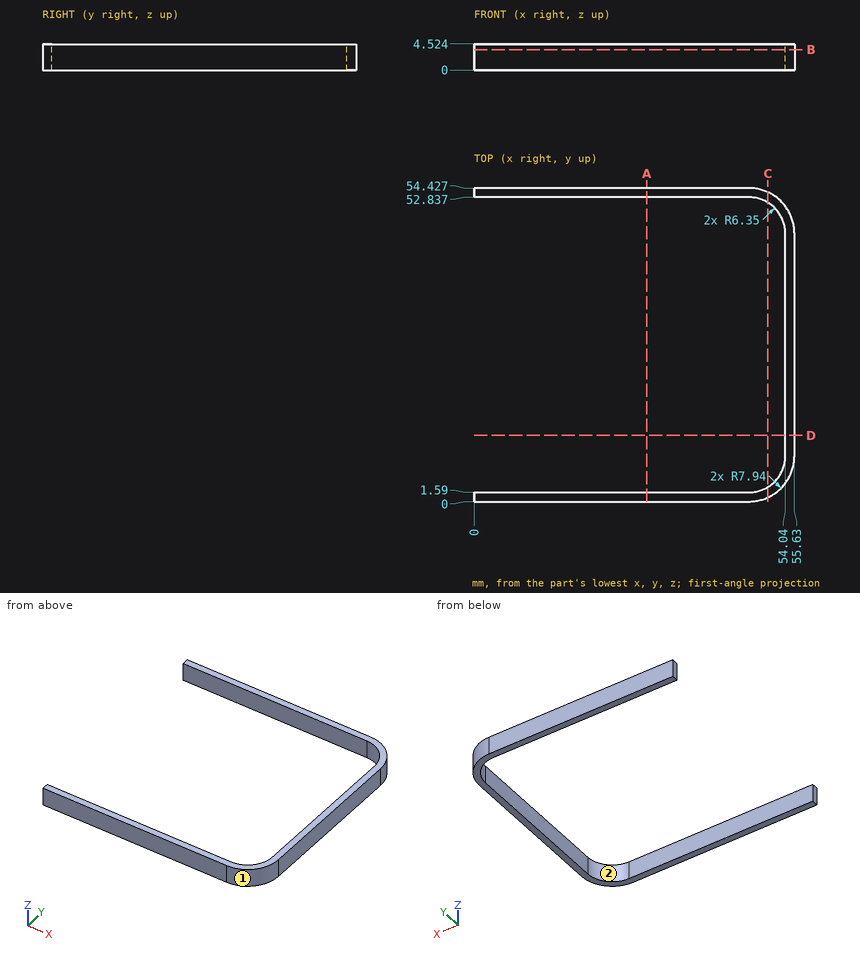
Design review of the part shown in the three views and the two pictorial views. Dimensions are in mm from the part's minimum x, y and z. Give positions to 0.01 mm unless a question says otherwise; leave off trailing zeros. Loops run counter-clockwise (first coordinate to the right, second up) from the corner with the lowest first, then second, coordinate; pieces in that order, holes last. Notation, with made-up numbers: M -27,-37 L -7,-37 A25 cw -7,-11 Z; hole C 12,12 d4. An arc over 180 degrees is marked long. Answer as a JSON object with one key per item and string values.
Item 1: We need section B-B (z = 3.55). State the section outline as (x, y) points.
Output values:
{"outline": "M 0,0 L 47.69,0 A7.94 ccw 55.63,7.94 L 55.63,46.49 A7.94 ccw 47.69,54.43 L 0,54.43 L 0,52.84 L 47.69,52.84 A6.35 cw 54.04,46.49 L 54.04,7.94 A6.35 cw 47.69,1.59 L 0,1.59 Z"}
Item 2: For P1, Ø2.5, axis at x = 14.5, z = 3, coming from the -Y side, flat-tipped, find the tip position at first contact; note if it passes through.
Output values:
{"P1": "stops at y = 0"}
Item 3: Mouldability with a two-part tool opening along Y and no side actions: class the marked faces 1 and 2 as pulls with the +Y half, pulls with the -Y half, needs draft (parallel to the pull), parting line crosses it, or undercut.
Output values:
{"face 1": "pulls with the -Y half", "face 2": "undercut"}
Item 4: We need section D-D (y = 11.5). State the section outline as (x, z) points.
Output values:
{"outline": "M 54.04,0 L 55.63,0 L 55.63,4.52 L 54.04,4.52 Z"}
Item 5: We need section A-A (x = 30). State the section outline as (y, z) points.
Output values:
{"outline": "M 0,0 L 1.59,0 L 1.59,4.52 L 0,4.52 Z; M 52.84,0 L 54.43,0 L 54.43,4.52 L 52.84,4.52 Z"}
Item 6: Wall thickness on line 1 along Y through (x, z) = (8.5, 2.3); line 2 along X through (y, z) = (43, 1.5); line 3 along Y through (x, z) = (49, 1.7): over which ranges is each line inside the solid? List them lowest first.
Output values:
{"line 1": "y = 0 to 1.59, 52.84 to 54.43", "line 2": "x = 54.04 to 55.63", "line 3": "y = 0.11 to 1.73, 52.7 to 54.32"}
Item 7: We need section C-C (x = 51). State the section outline as (y, z) points.
Output values:
{"outline": "M 0.72,0 L 2.52,0 L 2.52,4.52 L 0.72,4.52 Z; M 51.91,0 L 53.7,0 L 53.7,4.52 L 51.91,4.52 Z"}
